from build123d import *

# Parameters (mm, degrees)
F0_W     = 304.8
F0_H     = 1473.2
F1_DEPTH = 317.5
F2_T     = -3.175
F3_W     = 685.8
F3_H     = 1524
F3_W_2   = 628.65
F3_H_2   = 1466.85
F4_DEPTH = 3.175
F5_W     = 508
F5_H     = 203.2
F6_DEPTH = 304.801
F7_W     = 508
F7_H     = 203.2
F8_DEPTH = 3.175


with BuildPart() as f1:
    # F0 (on Right) → F1 (new body, symmetric)
    with BuildSketch(Plane.YZ):
        Rectangle(F0_W, F0_H)
    extrude(amount=F1_DEPTH, both=True)

    # F2
    f2_openings = [f1.faces().sort_by_distance(p)[0] for p in [
        (0, -152.4, 0),
    ]]
    offset(amount=F2_T, openings=f2_openings)

    # F3 (on face) → F4 (join)
    with BuildSketch(Plane.XZ.offset(152.4)):
        Rectangle(F3_W, F3_H)
        Rectangle(F3_W_2, F3_H_2, mode=Mode.SUBTRACT)
    extrude(amount=-F4_DEPTH)

    # F5 (on face) → F6 (cut, through all)
    with BuildSketch(Plane(origin=(0, 152.4, 0), x_dir=(-1, 0, 0), z_dir=(0, 1, 0))):
        with Locations((0, 584.2)):
            Rectangle(F5_W, F5_H)
    extrude(amount=-F6_DEPTH, mode=Mode.SUBTRACT)

    # F7 (on face) → F8 (cut, through all)
    with BuildSketch(Plane(origin=(0, 0, -736.6), x_dir=(1, 0, 0), z_dir=(0, 0, -1))):
        Rectangle(F7_W, F7_H)
    extrude(amount=-F8_DEPTH, mode=Mode.SUBTRACT)


solid = f1.part
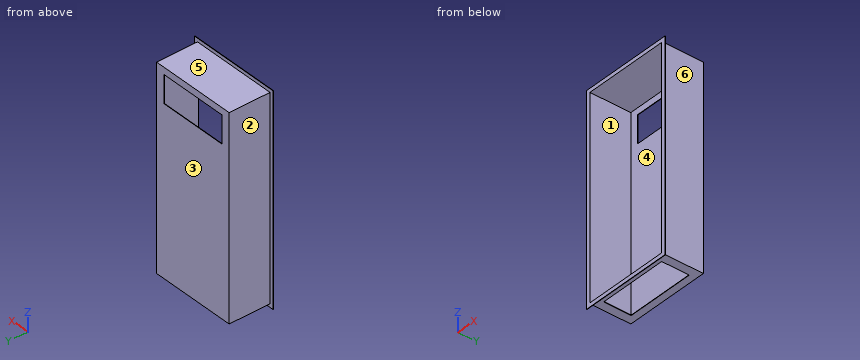
For this review, take the finished solid that the model builds, in its own axes (mm). Face numbers are marked on the shaded views. A direction names the side the tool comes from. Coordinates: 2 decimals unless noted, no trailing zeros. Loops run counter-clockwise (first coordinate to the right, second up) from the corner with the lowest first, then second, coordinate; pieces in that order, holes last. Notation, with made-up numbers: (-1.5, 3.5) - (26.5, 3.5) arc R15 ccw to (26.5, 19.5) - close; hole circle Ø4 at (75, 85). An arc over 180 degrees is marked (long way). Use a Markdown table: item, result. Add a question column.
Item 1: We need section B-B (x = -239.5). Give the boundary of the cut face in (y, z) (3 decimals), and give its area (3 significant figures).
Item 2: Insertion check: pin 1 Ø1.6 at (y, z) = (151.5, 544) entering from -X; pin 2 Ø5 at (x, z) = (225, 134.5) entering from -Y (3 decimals); pin 3 Ø3.5 at (y, z) = (-48.5, -736) entering from +X. Each pin has a flat end and moves straight along its axis. Give the tip position at first contact, or say it passes through.
Item 3: Tool access review of the marked faces 4, 5 and 6: name each direction out of +Z, -Z, +X, -X, +Y, -Y from which nothing blocks a thin tool from reaching the whole face with its end or side.
Item 4: We need section C-C (z = 154). Give the boundary of the cut face in (x, y) (3 decimals).
Item 5: For line 1 (X direction, y = -129, z = -203.5) (3 decimals); line 2 (Z direction, x = -272, y = -27) (3 decimals); line 3 (Y direction, x = 40.5, z = -364) (3 decimals), list the stretches that pass through material, from the lowest coordinate up.
Item 6: Mouldability with a two-part tool opening along X and no side actions: class the marked faces 1, 2 and 3 as pulls with the +X half, pulls with the -X half, needs draft (parallel to the pull), parting line crosses it, or undercut.
Item 7: We need section A-A (y = 116.5). Give the boundary of the cut face in (x, z) (3 decimals).
Results list:
| question | item | result |
|---|---|---|
| 1 | outline | (-152.4, -762) - (-149.225, -762) - (-149.225, -736.6) - (-101.6, -736.6) - (-101.6, -733.425) - (-152.4, -733.425) - close; (-152.4, 733.425) - (149.225, 733.425) - (149.225, 685.8) - (152.4, 685.8) - (152.4, 736.6) - (-149.225, 736.6) - (-149.225, 762) - (-152.4, 762) - close; (101.6, -736.6) - (152.4, -736.6) - (152.4, 482.6) - (149.225, 482.6) - (149.225, -733.425) - (101.6, -733.425) - close |
| 1 | area | 5,460 mm^2 |
| 2 | pin 1 | stops at x = -317.5 |
| 2 | pin 2 | stops at y = 149.225 |
| 2 | pin 3 | stops at x = 317.5 |
| 3 | face 4 | -Y |
| 3 | face 5 | +Z, +X, -X, +Y |
| 3 | face 6 | +Z, -Z, +X, +Y |
| 4 | outline | (-342.9, -152.4) - (-314.325, -152.4) - (-314.325, 149.225) - (314.325, 149.225) - (314.325, -152.4) - (342.9, -152.4) - (342.9, -149.225) - (317.5, -149.225) - (317.5, 152.4) - (-317.5, 152.4) - (-317.5, -149.225) - (-342.9, -149.225) - close |
| 5 | line 1 | x = -317.5 to -314.325, 314.325 to 317.5 |
| 5 | line 2 | z = -736.6 to -733.425, 733.425 to 736.6 |
| 5 | line 3 | y = 149.225 to 152.4 |
| 6 | face 1 | undercut |
| 6 | face 2 | pulls with the -X half |
| 6 | face 3 | needs draft |
| 7 | outline | (-317.5, -736.6) - (317.5, -736.6) - (317.5, 736.6) - (-317.5, 736.6) - close; hole (-314.325, -733.425) - (314.325, -733.425) - (314.325, 733.425) - (-314.325, 733.425) - close |
